Part print with two shaded views. Sizes in mm from the minimum x, y, z corner. Round coordinates to 2 decimals unless told otherwise and drop trailing zeros. Loops run counter-clockwise (first coordinate to the right, second up) from the corner with the lowest first, then second, coordinate; pieces in that order, holes last. Notation, with made-up numbers: (68.25, 59) - (102.25, 59) arc R18 ccw to (102.25, 64) - close; hole circle Ø3 at (75.5, 12). An arc over 180 degrees is marked (long way). Write each question's results on one line, items separated by ' | '. Start each with the question number.
(1) Cut at D-D, the plane y = 7.5. List the corners of the cut face in (x, z) (1 decimal).
(2) Flat gauge pins, fed straight in: P1, Ø2, axis at x = 8.5, y = 26, coming from the -Z side; P2, Ø0.5, axis at x = 10.5, z = 0.5, coming from the +Y side. Where does each tip first touch, or does it go through?
(3) Cut at C-C, the plane x = 10.75. List the corners of the cut face in (y, z).
(4) Cut at A-A, the plane y = 30. List the corners of the cut face in (x, z).
(5) Drill centre lines: L1, parallel to Y at x = 5.75, z = 0.8; L2, parallel to X at y = 4.5, z = 0.7 (1 decimal); L3, parallel to Y at x = 17.5, z = 0.8 (1 decimal). Where is each one in solid material? Low to high.
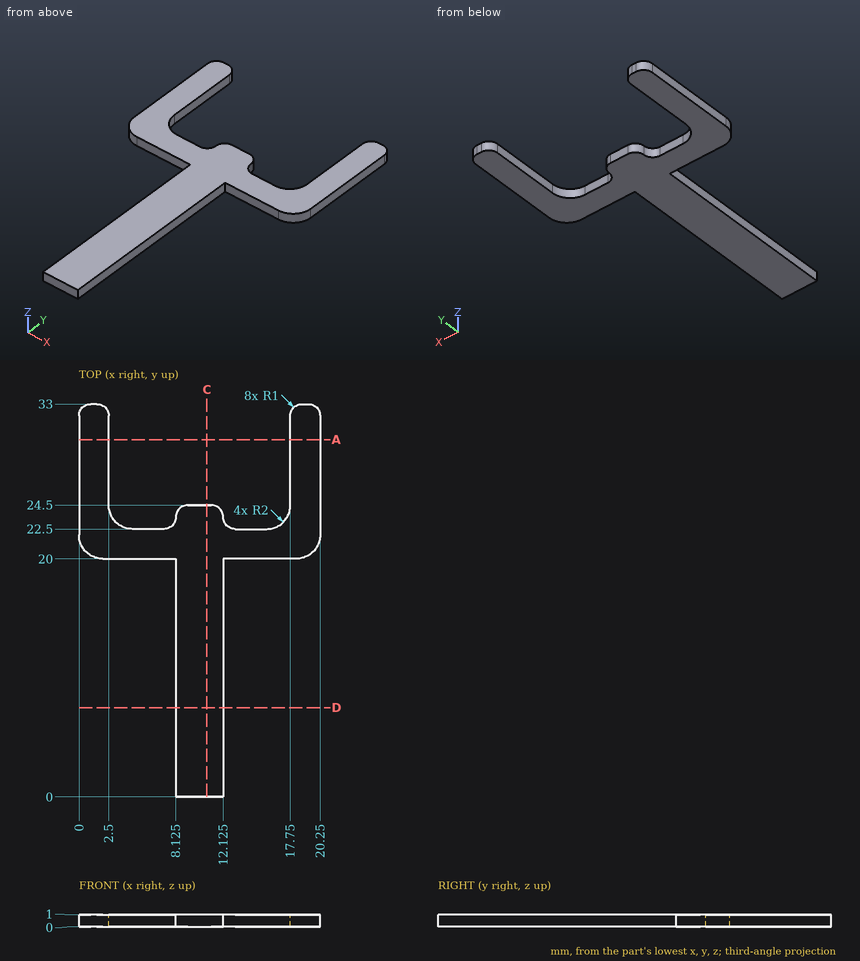
A:
1) outline: (8.1, 0) - (12.1, 0) - (12.1, 1) - (8.1, 1) - close
2) P1: through | P2: y = 24.5
3) outline: (0, 0) - (24.5, 0) - (24.5, 1) - (0, 1) - close
4) outline: (0, 0) - (2.5, 0) - (2.5, 1) - (0, 1) - close; (17.75, 0) - (20.25, 0) - (20.25, 1) - (17.75, 1) - close
5) L1: 20 to 22.5 | L2: 8.1 to 12.1 | L3: 20 to 23.5
